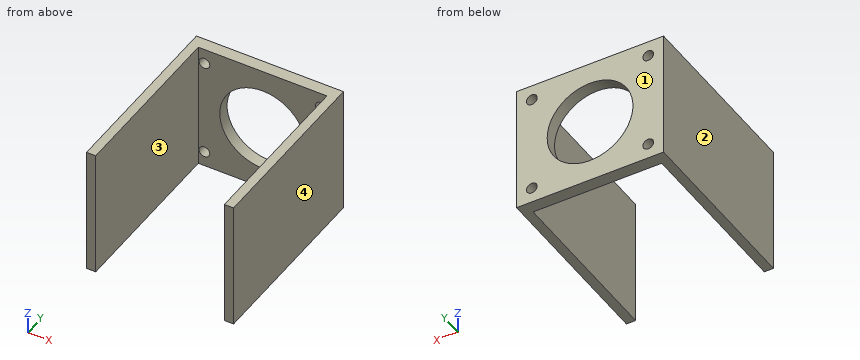
```python
from build123d import *

# Parameters (mm, degrees)
BOSS_EXTRUDE1_DEPTH = 42
SKETCH2_R           = 1.75
SKETCH2_R_2         = 14
CUT_EXTRUDE1_DEPTH  = 61


with BuildPart() as part:
    # Sketch1 → Boss-Extrude1 (new body)
    with BuildSketch(Plane.XY):
        Polygon((-21, -30), (-21, 26), (21, 26), (21, -30), (24, -30), (24, 30), (-24, 30), (-24, -30), align=None)
    extrude(amount=BOSS_EXTRUDE1_DEPTH)

    # Sketch2 → Cut-Extrude1 (cut, through all)
    with BuildSketch(Plane(origin=(0, 30, 0), x_dir=(1, 0, 0), z_dir=(0, 1, 0))):
        with Locations((19, -37)):
            Circle(SKETCH2_R)
        with Locations((19, -5)):
            Circle(SKETCH2_R)
        with Locations((-19, -37)):
            Circle(SKETCH2_R)
        with Locations((-19, -5)):
            Circle(SKETCH2_R)
        with Locations((0, -21)):
            Circle(SKETCH2_R_2)
    extrude(amount=-CUT_EXTRUDE1_DEPTH, mode=Mode.SUBTRACT)


solid = part.part
```
Here's how the part is built. I have some questions about the finished solid (model axes, mm). Face numbers are marked on the shaded views. Coordinates: 2 decimals unless noted, no trailing zeros. Write each loop counter-clockwise with the first axis right and the second up, starting at its lowest first coordinate (ties: lowest second). Pieces come first, ordered by that corner, then holes. Notation, with made-up numbers: M 20,69 L 77,69 A15 cw 77,89 Z; hole C 62.25,-5 d4. An arc over 180 degrees is marked long. Answer as CSV lines item,"result". Start each with the question number.
Q1. Suppose I cut it at B-B, the plane x = 0. List the corners of the cut face in (y, z) for me, then the cut area to 3 significant figures.
Q2. Will these pins go through, and if not, where does the flat tip stop? pin 1 Ø3 at (x, z) = (-19, 37) entering from -Y; pin 2 Ø3 at (x, z) = (-18, 37) entering from -Y.
Q3. Suppose I cut it at C-C, the plane y = -26. List the corners of the cut face in (x, z) for me, then the cut area to 3 significant figures.
Q4. If we mould it in two halves opening along X, with no side actions, what happens to the marked faces 1, 2, 3 and 4? For each: pulls with the +X half, pulls with the -X half, needs draft (parallel to the pull), parting line crosses it, or undercut.
Q5. Suppose I cut it at D-D, the plane x = 19. List the corners of the cut face in (y, z) for me, then the cut area to 3 significant figures.
Q6. I need wall thicknesses on probe 1 along X at (y, z) = (28, 5); probe 2 along Z at (x, y) = (19, 27); probe 3 along X at (y, z) = (-1, 33). Which ranges of each line are inside material? Lowest first, please. Write a range as [from, to].
Q7. Suppose I cut it at A-A, the plane z = 37. List the corners of the cut face in (x, y) for me, then the cut area to 3 significant figures.
Entries:
1,outline,"M 26,0 L 30,0 L 30,7 L 26,7 Z; M 26,35 L 30,35 L 30,42 L 26,42 Z"
1,area,"56.0 mm²"
2,pin 1,"passes through"
2,pin 2,"stops at y = 26"
3,outline,"M -24,0 L -21,0 L -21,42 L -24,42 Z; M 21,0 L 24,0 L 24,42 L 21,42 Z"
3,area,"252 mm²"
4,face 1,"needs draft"
4,face 2,"pulls with the -X half"
4,face 3,"undercut"
4,face 4,"pulls with the +X half"
5,outline,"M 26,0 L 30,0 L 30,3.25 L 26,3.25 Z; M 26,6.75 L 30,6.75 L 30,35.25 L 26,35.25 Z; M 26,38.75 L 30,38.75 L 30,42 L 26,42 Z"
5,area,"140 mm²"
6,probe 1,"x = [-24, -20.75], [-17.25, 17.25], [20.75, 24]"
6,probe 2,"z = [0, 3.25], [6.75, 35.25], [38.75, 42]"
6,probe 3,"x = [-24, -21], [21, 24]"
7,outline,"M -24,-30 L -21,-30 L -21,26 L -20.75,26 L -20.75,30 L -24,30 Z; M -17.25,26 L 17.25,26 L 17.25,30 L -17.25,30 Z; M 20.75,26 L 21,26 L 21,-30 L 24,-30 L 24,30 L 20.75,30 Z"
7,area,"500 mm²"
